Here's how the part is built. I have some questions about the finished solid (model axes, mm). Face numbers are marked on the shaded views. Round coordinates to 2 decimals unless told otherwise and drop trailing zeros. Write each loop counter-clockwise with the first axis right and the second up, starting at its lowest first coordinate (ties: lowest second). Pieces come first, ordered by that corner, then holes. Notation, with made-up numbers: (19.5, -24.75) - (67.5, -24.75) arc R17 cw to (67.5, -2.75) - close; hole circle Ø10 at (6, 31.5). An arc over 180 degrees is marked (long way). Return JSON: item names as keys, results as strings. Group by question number.
```python
from build123d import *
from build123d.topology import SkipClean

# Parameters (mm, degrees)
SKETCH1_R             = 28.5
SKETCH1_R_2           = 27.5
BOSS_EXTRUDE1_DEPTH   = 15
SKETCH1_R_3           = 23.5
SKETCH1_R_4           = 22.5
BOSS_EXTRUDE1_2_DEPTH = 15
CUT_EXTRUDE2_DEPTH    = 5
BOSS_EXTRUDE3_DEPTH   = 2
SKETCH5_R             = 1.25
BOSS_EXTRUDE4_DEPTH   = 6
CUT_EXTRUDE3_START    = -2
CUT_EXTRUDE3_DEPTH    = 2
SKETCH7_W             = 2.5
SKETCH7_H             = 1.5
BOSS_EXTRUDE5_DEPTH   = 5
CIRPATTERN1_COUNT     = 5


with BuildPart() as part:
    # Sketch1 → Boss-Extrude1 (new body)
    with BuildSketch(Plane(origin=(0, 0, 0), x_dir=(1, 0, 0), z_dir=(0, 1, 0))):
        with Locations(Location((0, 0, 0), (0, 0, 270))):
            Circle(SKETCH1_R)
        with Locations(Location((0, 0, 0), (0, 0, 270))):
            Circle(SKETCH1_R_2, mode=Mode.SUBTRACT)
    extrude(amount=BOSS_EXTRUDE1_DEPTH)



with BuildPart() as body_2:
    # Sketch1 → Boss-Extrude1 2 (new body)
    with BuildSketch(Plane(origin=(0, 0, 0), x_dir=(1, 0, 0), z_dir=(0, 1, 0))):
        with Locations(Location((0, 0, 0), (0, 0, 270))):
            Circle(SKETCH1_R_3)
        with Locations(Location((0, 0, 0), (0, 0, 270))):
            Circle(SKETCH1_R_4, mode=Mode.SUBTRACT)
    extrude(amount=BOSS_EXTRUDE1_2_DEPTH)

    # Sketch4 → Cut-Extrude2 (cut)
    with BuildSketch(Plane(origin=(0, 4, 0), x_dir=(-1, 0, 0), z_dir=(0, -1, 0))):
        with BuildLine():
            Line((22.912407012, 5.222222222), (21.937410968, 5))
            ThreePointArc((21.937410968, 5), (22.5, 0), (21.937410968, -5))
            Line((21.937410968, -5), (22.912407012, -5.222222222))
            ThreePointArc((22.912407012, -5.222222222), (23.5, 0), (22.912407012, 5.222222222))
        make_face()
        with BuildLine():
            Line((-22.912407012, -5.222222222), (-21.937410968, -5))
            ThreePointArc((-21.937410968, -5), (-22.5, 0), (-21.937410968, 5))
            Line((-21.937410968, 5), (-22.912407012, 5.222222222))
            ThreePointArc((-22.912407012, 5.222222222), (-23.5, 0), (-22.912407012, -5.222222222))
        make_face()
        with BuildLine():
            Line((-5.222222222, -22.912407012), (-5, -21.937410968))
            ThreePointArc((-5, -21.937410968), (0, -22.5), (5, -21.937410968))
            Line((5, -21.937410968), (5.222222222, -22.912407012))
            ThreePointArc((5.222222222, -22.912407012), (0, -23.5), (-5.222222222, -22.912407012))
        make_face()
    extrude(amount=-CUT_EXTRUDE2_DEPTH, mode=Mode.SUBTRACT)


with BuildPart() as part_1:
    with SkipClean():  # the faces are left unmerged after this step: merging them gives an invalid solid
        add(part.part)

        add(body_2.part)  # Boss-Extrude3 merges body 2
        # Sketch3 → Boss-Extrude3 (add)
        with BuildSketch(Plane(origin=(0, 15, 0), x_dir=(1, 0, 0), z_dir=(0, 1, 0))):
            with BuildLine():
                Line((-28.5, 0), (28.5, 0))
                ThreePointArc((28.5, 0), (0, -28.5), (-28.5, 0))
            make_face()
        extrude(amount=BOSS_EXTRUDE3_DEPTH)
    add(part_1.part.scale(1), mode=Mode.REPLACE)  # the faces are merged on a copy

    # Sketch5 → Boss-Extrude4 (add)
    with BuildSketch(Plane(origin=(0, 17, 0), x_dir=(1, 0, 0), z_dir=(0, 1, 0))):
        with Locations(Location((0, -3.253176926, 0), (0, 0, 270))):
            Circle(SKETCH5_R)
    extrude(amount=BOSS_EXTRUDE4_DEPTH)

    # Sketch6 → Cut-Extrude3 (cut)
    with BuildSketch(Plane(origin=(0, 17, 0), x_dir=(1, 0, 0), z_dir=(0, 1, 0)).offset(CUT_EXTRUDE3_START)):
        with BuildLine():
            Line((-27.941794444, -5.613031555), (27.941794444, -5.613031555))
            ThreePointArc((27.941794444, -5.613031555), (0, -28.5), (-27.941794444, -5.613031555))
        make_face()
    extrude(amount=CUT_EXTRUDE3_DEPTH, mode=Mode.SUBTRACT)

    # Sketch7 → Boss-Extrude5 (add)
    with BuildSketch(Plane.XZ):
        with Locations((0, -21.75)):
            Rectangle(SKETCH7_W, SKETCH7_H)
    boss_extrude5 = extrude(amount=-BOSS_EXTRUDE5_DEPTH)

    # CirPattern1: Boss-Extrude5 ×5 about axis
    cirpattern1_axis = Axis((0, 0, 0), (0, 1, 0))
    for i in range(1, CIRPATTERN1_COUNT):
        add(boss_extrude5.rotate(cirpattern1_axis, i * 360 / CIRPATTERN1_COUNT))


solid = part_1.part
```
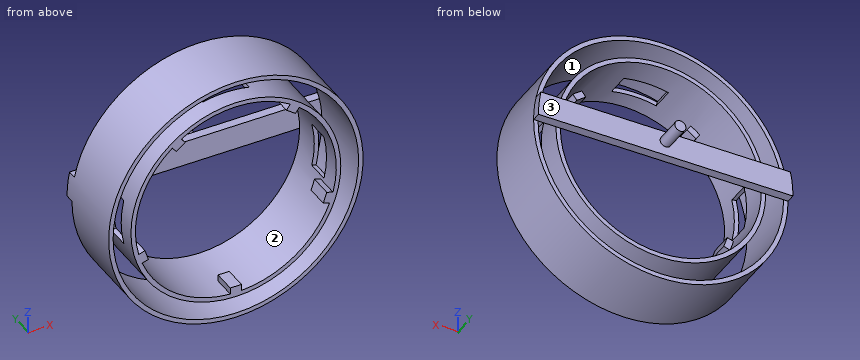
1) Imagine slicing it at A-A (y = 3). Please give me the cut outline in (x, z), plus the area to 3 significant figures.
2) Imagine slicing it at C-C (z = -18.5). Please give me the cut outline in (x, y).
3) Will these pins go through, and if not, where does the flat tip stop? pin 1 Ø2 at (x, y) = (8.5, 15.5) entering from -Z; pin 2 Ø1.1 at (x, z) = (21, -6.5) entering from +Y; pin 3 Ø10 at (y, z) = (14, 3) entering from +X; pin 4 Ø1.5 at (x, y) = (-11.5, 3.5) entering from -Z.
4) Imagine slicing it at D-D (x = 17.5). Please give me the cut outline in (y, z), plus the area to 3 significant figures.
5) I need wall thicknesses on line 1 along Z through (x, y) = (0, 10); line 2 along Z through (x, y) = (0, 6). Which ranges of each line are inside material? Lowest first, please.
6) If we mould it in two halves opening along X, with no side actions, what happens to the marked faces 1, 2 and 3? For each: released by +X, released by -X, zero draft, split by the parting line, or undercut.
7) Imagine slicing it at B-B (x = 0). Give the number of separate pieces and of enclosed holes in the cut face, plus the area to 3 significant figures.
Results found:
{
 "1": {"outline": "circle Ø57 at (0, 0); circle Ø47 at (0, 0); hole circle Ø55 at (0, 0); hole (-21.75, -5.75) - (-20.36, -5.3) - (-19.59, -7.68) - (-20.98, -8.13) arc R22.5 ccw to (-1.25, -22.47) - (-1.25, -21) - (1.25, -21) - (1.25, -22.47) arc R22.5 ccw to (20.98, -8.13) - (19.59, -7.68) - (20.36, -5.3) - (21.75, -5.75) arc R22.5 ccw to (14.22, 17.44) - (13.35, 16.25) - (11.33, 17.72) - (12.19, 18.91) arc R22.5 ccw to (-12.19, 18.91) - (-11.33, 17.72) - (-13.35, 16.25) - (-14.22, 17.44) arc R22.5 ccw to start", "area": "339 mm²"},
 "2": {"outline": "(-21.68, 0) - (-20.35, 0) - (-20.35, 15) - (-21.68, 15) - close; (-14.49, 0) - (-12.81, 0) - (-12.81, 15) - (-14.49, 15) - close; (12.81, 0) - (14.49, 0) - (14.49, 15) - (12.81, 15) - close; (20.35, 0) - (21.68, 0) - (21.68, 15) - (20.35, 15) - close"},
 "3": {"pin 1": "stops at z = -27.46", "pin 2": "stops at y = 15", "pin 3": "stops at x = 28.5", "pin 4": "stops at z = -26.39"},
 "4": {"outline": "(0, -22.49) - (15, -22.49) - (15, -21.21) - (0, -21.21) - close; (0, -15.68) - (15, -15.68) - (15, -14.14) - (0, -14.14) - close; (0, 14.14) - (15, 14.14) - (15, 15.68) - (0, 15.68) - close; (0, 21.21) - (15, 21.21) - (15, 22.49) - (0, 22.49) - close; (15, 0) - (17, 0) - (17, 5.61) - (15, 5.61) - close", "area": "95.9 mm²"},
 "5": {"line 1": "z = -28.5 to -27.5, -23.5 to -22.5, 22.5 to 23.5, 27.5 to 28.5", "line 2": "z = -28.5 to -27.5, -23.5 to -22.5, 27.5 to 28.5"},
 "6": {"face 1": "undercut", "face 2": "undercut", "face 3": "zero draft"},
 "7": {"separate pieces": "6", "enclosed holes": "0", "area": "88.7 mm²"}
}
